```python
from build123d import *

# Parameters (mm, degrees)
SKETCH1_W      = 76.2
SKETCH1_H      = 9.525
EXTRUDE1_DEPTH = 6.35


with BuildPart() as part:
    # Sketch1 → Extrude1 (new body)
    with BuildSketch(Plane.XY):
        with BuildLine():
            Line((47.625, -59.874659688), (47.625, -105.430018939))
            ThreePointArc((47.625, -105.430018939), (44.835192091, -112.16521103), (38.1, -114.955018939))
            Line((38.1, -114.955018939), (-38.1, -114.955018939))
            ThreePointArc((-38.1, -114.955018939), (-44.835192091, -112.16521103), (-47.625, -105.430018939))
            Line((-47.625, -105.430018939), (-47.625, -61.523712718))
            ThreePointArc((-47.625, -61.523712718), (-31.103765958, -19.76273177), (-37.103282828, 24.744981061))
            ThreePointArc((-37.103282828, 24.744981061), (0, 61.848263889), (37.103282828, 24.744981061))
            ThreePointArc((37.103282828, 24.744981061), (31.556422492, -18.908685267), (47.625, -59.874659688))
        make_face()
        with BuildLine():
            Line((-9.520105929, -57.499718912), (-9.520105929, -8.508405033))
            ThreePointArc((-9.520105929, -8.508405033), (-9.524795338, -8.354131878), (-9.538846249, -8.200428368))
            ThreePointArc((-9.538846249, -8.200428368), (-12.897895618, 8.373789137), (-18.804224779, 24.220024477))
            ThreePointArc((-18.804224779, 24.220024477), (-18.98980734, 24.783579345), (-19.039585391, 25.374812905))
            ThreePointArc((-19.039585391, 25.374812905), (0.000886222, 43.79498104), (19.039643909, 25.373041427))
            ThreePointArc((19.039643909, 25.373041427), (18.990133662, 24.783398196), (18.805538674, 24.221210421))
            ThreePointArc((18.805538674, 24.221210421), (12.876614575, 8.222405207), (9.542532972, -8.510729859))
            ThreePointArc((9.542532972, -8.510729859), (9.529387032, -8.65943529), (9.525, -8.808656182))
            Line((9.525, -8.808656182), (9.525, -57.805018939))
            ThreePointArc((9.525, -57.805018939), (-0.152669626, -67.328795343), (-9.520105929, -57.499718912))
        make_face(mode=Mode.SUBTRACT)
        with Locations((1.633712121, -100.667518939)):
            Rectangle(SKETCH1_W, SKETCH1_H, mode=Mode.SUBTRACT)
    extrude(amount=EXTRUDE1_DEPTH)


solid = part.part
```
Design review of the part built by this model. Coordinates are the model's own, in mm. A direction names the side the tool comes from. Give positions to 0.01 mm unless a question says otherwise; leave off trailing zeros. Write each loop counter-clockwise with the first axis right and the second up, starting at its lowest first coordinate (ties: lowest second). Pieces come first, ordered by that corner, then holes. Notation, with made-up numbers: (22, 82.5) -> (52, 82.5) arc R24 cw to (52, 101.5) -> close; hole circle Ø1 at (-1.5, 40). An arc over 180 degrees is marked (long way). Answer in a Markdown table with one row per item.
(1) Consider section C-C (z = 3.5). State the section outline as (x, y) points (3 decimals), then the cut area to 3 significant figures.
Results:
| item | result |
|---|---|
| outline | (-47.625, -105.43) arc R9.525 ccw to (-38.1, -114.955) -> (38.1, -114.955) arc R9.525 ccw to (47.625, -105.43) -> (47.625, -59.875) arc R88.9 cw to (37.103, 24.745) arc R37.103 ccw to (-37.103, 24.745) arc R88.9 cw to (-47.625, -61.524) -> close; hole (-36.466, -105.43) -> (39.734, -105.43) -> (39.734, -95.905) -> (-36.466, -95.905) -> close; hole (-19.04, 25.375) arc R2.54 ccw to (-18.804, 24.22) arc R107.95 cw to (-9.539, -8.2) arc R2.54 cw to (-9.52, -8.508) -> (-9.52, -57.5) arc R9.525 ccw (long way) to (9.525, -57.805) -> (9.525, -8.809) arc R2.54 cw to (9.543, -8.511) arc R107.95 cw to (18.806, 24.221) arc R2.54 ccw to (19.04, 25.373) arc R19.05 ccw to start |
| area | 9,970 mm2 |
(2) Consider section A-A (x = 0). State the section outline as (y, z) points, then the cut area to 3 significant figures.
Results:
| item | result |
|---|---|
| outline | (-114.96, 0) -> (-105.43, 0) -> (-105.43, 6.35) -> (-114.96, 6.35) -> close; (-95.91, 0) -> (-67.33, 0) -> (-67.33, 6.35) -> (-95.91, 6.35) -> close; (43.79, 0) -> (61.85, 0) -> (61.85, 6.35) -> (43.79, 6.35) -> close |
| area | 357 mm2 |
(3) Consider section B-B (y = -50.5). State the section outline as (x, z) points (3 decimals), then the cut area to 3 significant figures.
Results:
| item | result |
|---|---|
| outline | (-40.731, 0) -> (-9.52, 0) -> (-9.52, 6.35) -> (-40.731, 6.35) -> close; (9.525, 0) -> (41.727, 0) -> (41.727, 6.35) -> (9.525, 6.35) -> close |
| area | 403 mm2 |
(4) For faces 1 (the cylindrical face through (-31.183, -20.393, 3.131)), 2 (the flat face through (1, -95.905, 3)), list the 3-axis set-ups (+Z, -Z, +X, -X, +Y, -Y) from which the entire face can be reached by the end or side of a thin tool; tool diameter is ignored.
Results:
| item | result |
|---|---|
| face 1 | +Z, -Z, -X |
| face 2 | +Z, -Z |
(5) Clearance check with a flat-ended pin moving along its axis: pin 1 (3 mm diameter, centred on y = -24.5, z = 4.5, fed in from +X). State where the tip first meets the part, or that it passes through.
Results:
| item | result |
|---|---|
| pin 1 | x = 32.73 |
(6) Mouldability with a two-part tool opening along X and no side actions: class faces 3 (the flat face through (1, -114.955, 3)), 4 (the flat face through (1, -105.43, 3)), 5 (the cylindrical face through (31.48, -18.29, 3.13)), 6 (the flat face through (-47.625, -84, 3)) as +X half, -X half, draft (parallel to the pull), parting line (faces both ways), or undercut.
Results:
| item | result |
|---|---|
| face 3 | draft |
| face 4 | undercut |
| face 5 | +X half |
| face 6 | -X half |
(7) Consider section D-D (y = -27.5). State the section outline as (x, z) points (3 decimals), then the cut area to 3 significant figures.
Results:
| item | result |
|---|---|
| outline | (-32.396, 0) -> (-9.52, 0) -> (-9.52, 6.35) -> (-32.396, 6.35) -> close; (9.525, 0) -> (33.056, 0) -> (33.056, 6.35) -> (9.525, 6.35) -> close |
| area | 295 mm2 |
(8) To check wall thickness, follow probe 1 along X at (y, z) = (-99, 6.25) (3 decimals); probe 2 along Y at (x, z) = (-8.5, 5.5); probe 3 along Y at (x, z) = (-5, 2.5). State the ranges of each line that lie inside material, in increasing order.
Results:
| item | result |
|---|---|
| probe 1 | -47.625 to -36.466, 39.734 to 47.625 |
| probe 2 | -114.96 to -105.43, -95.91 to -62.1, 41.79 to 60.86 |
| probe 3 | -114.96 to -105.43, -95.91 to -65.91, 43.13 to 61.51 |
